Build history of the part. All positions in model axes, mm. Face numbers are marked on the shaded views. A direction names the side the tool comes from. Give positions to 0.01 mm unless a question says otherwise; leave off trailing zeros. Loops run counter-clockwise (first coordinate to the right, second up) from the corner with the lowest first, then second, coordinate; pieces in that order, holes last.
1) Band-saw the part on C-C on z = 32. List the corners of the cut face in (x, y), then the cut area to 3 significant figures.
2) Wall check: line 1 (Z direction, x = -1, y = 14) (1 decimal); line 2 (X direction, y = 10.16, z = 35.75); line 3 (Y direction, x = 0, z = 38). Give the ranges that are in metal, low to high.
3) Band-saw the part on B-B on x = -1. State how many separate pieces and enclosed holes the cut face has, then the cut area to 3 significant figures.
4) 3-axis set-ups, long thin cutter, end or side, ignore diameter. For the marked faces 1, 2 and 3: which of +Z, -Z, +X, -X, +Y, -Y reach the whole face in a straight line?
5) Two-plate mould, pull along Z, no slides. Class the marked faces 4, 5, 6 and 7: +Z half, -Z half, draft (parallel to the pull), parting line (faces both ways), or undercut.
6) Flat gauge pins, fed straight in: P1, Ø7.5, axis at x = 8.5, z = 36.5, coming from the +Y side; P2, Ø3, axis at x = -12, z = 5, coming from the -Y side. Where does each tip first touch, or does it go through?
7) Band-saw the part on D-D on z = 5. List the corners of the cut face in (x, y), then the cut area to 3 significant figures.
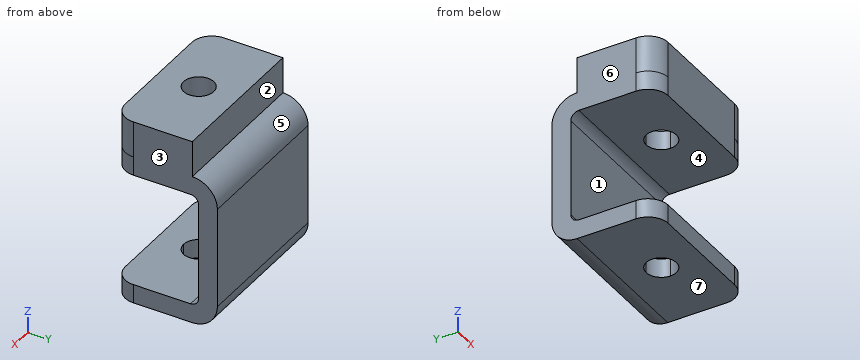
```python
from build123d import *

# Parameters (mm, degrees)
F1_DEPTH = 19.05
F3_DEPTH = 70.5358
F4_R     = 5.08
F5_R     = 3.81
F6_DEPTH = 9.144


with BuildPart() as f1:
    # F0 (on Right) → F1 (new body, symmetric)
    with BuildSketch(Plane.YZ):
        with BuildLine():
            Line((19.558, 0), (0, 0))
            Line((0, 0), (0, -4.7625))
            Line((0, -4.7625), (20.0025, -4.7625))
            ThreePointArc((20.0025, -4.7625), (24.492628, -2.902628), (26.3525, 1.5875))
            Line((26.3525, 1.5875), (26.3525, 26.9875))
            ThreePointArc((26.3525, 26.9875), (24.492628, 31.477628), (20.0025, 33.3375))
            Line((20.0025, 33.3375), (0, 33.3375))
            Line((0, 33.3375), (0, 28.575))
            Line((0, 28.575), (19.558, 28.575))
            ThreePointArc((19.558, 28.575), (20.994841, 27.979841), (21.59, 26.543))
            Line((21.59, 26.543), (21.59, 2.032))
            ThreePointArc((21.59, 2.032), (20.994841, 0.595159), (19.558, 0))
        make_face()
    extrude(amount=F1_DEPTH, both=True)

    # F2 (on face) → F3 (cut)
    with BuildSketch(Plane(origin=(0, 0, -4.7625), x_dir=(1, 0, 0), z_dir=(0, 0, -1))):
        with BuildLine():
            ThreePointArc((3.81, -10.16), (2.694077, -7.465923), (0, -6.35))
            Line((0, -6.35), (0, -13.97))
            ThreePointArc((0, -13.97), (2.694077, -12.854077), (3.81, -10.16))
        make_face()
        with BuildLine():
            Line((0, -13.97), (0, -6.35))
            ThreePointArc((0, -6.35), (-3.81, -10.16), (0, -13.97))
        make_face()
    extrude(amount=-F3_DEPTH, mode=Mode.SUBTRACT)

    # F4
    f4_edges = [f1.edges().sort_by_distance(p)[0] for p in [
        (-19.05, 0, 30.95625),
        (19.05, 0, 30.95625),
        (19.05, 0, -2.38125),
        (-19.05, 0, -2.38125),
    ]]
    fillet(f4_edges, radius=F4_R)

    # F5 (on face) → F6 (join)
    with BuildSketch(Plane.XY.offset(33.3375)):
        with BuildLine():
            Line((19.05, 20.0025), (-19.05, 20.0025))
            Line((-19.05, 20.0025), (-19.05, 5.08))
            ThreePointArc((-19.05, 5.08), (-17.562102, 1.487898), (-13.97, 0))
            Line((-13.97, 0), (13.97, 0))
            ThreePointArc((13.97, 0), (17.562102, 1.487898), (19.05, 5.08))
            Line((19.05, 5.08), (19.05, 20.0025))
        make_face()
        with Locations((0, 10.16)):
            Circle(F5_R, mode=Mode.SUBTRACT)
    extrude(amount=F6_DEPTH)


solid = f1.part
```
Findings below:
1. outline: (-19.05, 5.08) arc R5.08 ccw to (-13.97, 0) - (13.97, 0) arc R5.08 ccw to (19.05, 5.08) - (19.05, 23.9) - (-19.05, 23.9) - close; hole (0, 13.97) arc R3.81 ccw (long way) to (3.81, 10.16) arc R3.81 ccw to start
1. area: 854 mm2
2. line 1: z = -4.8 to 0, 28.6 to 42.5
2. line 2: x = -19.05 to -3.81, 3.81 to 19.05
2. line 3: y = 0 to 6.35, 13.97 to 20
3. separate pieces: 3
3. enclosed holes: 0
3. area: 417 mm2
4. face 1: +X, -X, -Y
4. face 2: +Z, +X, -X, +Y
4. face 3: +Z, -Z, +X, +Y, -Y
5. face 4: undercut
5. face 5: +Z half
5. face 6: draft
5. face 7: -Z half
6. P1: stops at y = 22.67
6. P2: stops at y = 21.59
7. outline: (-19.05, 21.59) - (19.05, 21.59) - (19.05, 26.35) - (-19.05, 26.35) - close
7. area: 181 mm2
